Part model, mm, in its own coordinate system. A direction names the side the tool comes from. Round coordinates to 2 decimals unless told otherwise and drop trailing zeros. Write each loop counter-clockwise with the first axis right and the second up, starting at its lowest first coordinate (ties: lowest second). Pieces come first, ordered by that corner, then holes. Notation, with made-up numbers: M 53.25,16 L 91.25,16 A27 cw 91.25,38 Z; hole C 49,-7 d7. An arc over 180 degrees is marked long. Answer as a JSON object with one key per item and string values. Group by question number.
1. Which spindle directions (+Z, -Z, +X, -X, +Y, -Y) get a long thin tool onto all of the face, cutting with end or side? Do faces 1 (the face through (-36, 6.9, 55)), 2 (the face through (36, 3.1, 30)), 3 (the face through (-29.35, 3.25, 41.67)), 4 (the face through (-36, 3.1, 51)). Say none if no direction does.
2. Drill centre lines: line 1 (Z direction, x = -23.5, y = 6.25); line 2 (Y direction, x = -29.5, z = 47); line 3 (X direction, y = 0.75, z = 6). Where is each one in solid material? Low to high. Write a range as from..to.
3. Two-plate mould, pull along Y, no slides. Class faces 5 (the face through (-1, 5, 60)), 6 (the face through (30.301, 7.805, 29.58)), 7 (the face through (-30.552, 2.387, 49.883)): +Y half, -Y half, draft (parallel to the pull), parting line (faces both ways), or undercut.
4. Drop flat-ended pins along their axis: pin 1 (0.5 mm diameter, centred on y = 0.5, z = 45.5, fed in from -X); pin 2 (8 mm diameter, centred on x = 34.5, z = 31.5, fed in from +Y); pin 3 (1.8 mm diameter, centred on x = -32.5, z = 48.5, fed in from +Y). Give the stop position or say it passes through.
5. Band-saw the part on A-A, the plane z = 30.5. Write the cut outline in (x, y), plus the area to 3 significant figures.
6. Band-saw the part on B-B, the plane y = 6. Write the cut outline in (x, z), plus the area to 3 significant figures.
7. Band-saw the part on D-D, the plane z = 53. Write the cut outline in (x, y).
8. Band-saw the part on C-C, the plane x = 34. Write the cut outline in (y, z).
from build123d import *

# Parameters (mm, degrees)
EXTRUDE_1_DEPTH     = 60
CUT_EXTRUDE_1_DEPTH = 17.3


with BuildPart() as part:
    # 스케치1 → 보스-돌출1 (new body)
    with BuildSketch(Plane.XY):
        with BuildLine():
            Line((29.8, 10), (-29.8, 10))
            Line((-29.8, 10), (-29.8, 9.4))
            ThreePointArc((-29.8, 9.4), (-30.532233047, 7.632233047), (-32.3, 6.9))
            Line((-32.3, 6.9), (-39.8, 6.9))
            Line((-39.8, 6.9), (-39.8, 3.1))
            Line((-39.8, 3.1), (-32.3, 3.1))
            ThreePointArc((-32.3, 3.1), (-30.532233047, 2.367766953), (-29.8, 0.6))
            Line((-29.8, 0.6), (-29.8, 0))
            Line((-29.8, 0), (29.8, 0))
            ThreePointArc((29.8, 0), (30.280633401, 2.170456935), (32.3, 3.1))
            Line((32.3, 3.1), (39.8, 3.1))
            Line((39.8, 3.1), (39.8, 6.9))
            Line((39.8, 6.9), (32.3, 6.9))
            ThreePointArc((32.3, 6.9), (30.280633401, 7.829543065), (29.8, 10))
        make_face()
    extrude(amount=EXTRUDE_1_DEPTH)

    # 스케치2 → 컷-돌출1 (cut)
    with BuildSketch(Plane.ZY.offset(39.8)):
        with BuildLine():
            Line((44, 4), (50, 4))
            Line((50, 4), (50, 8))
            Line((50, 8), (10, 8))
            Line((10, 8), (10, 4))
            Line((10, 4), (16, 4))
            ThreePointArc((16, 4), (18.828427125, 2.828427125), (20, 0))
            Line((20, 0), (40, 0))
            ThreePointArc((40, 0), (41.171572875, 2.828427125), (44, 4))
        make_face()
    extrude(amount=-CUT_EXTRUDE_1_DEPTH, mode=Mode.SUBTRACT)


solid = part.part
Worked answers:
{
 "1": {"face 1": "+Z, -Z, -X, +Y", "face 2": "+Z, -Z, +X, -Y", "face 3": "-X", "face 4": "+Z, -Z, -X, -Y"},
 "2": {"line 1": "z = 0..10, 50..60", "line 2": "y = 0..4, 8..10", "line 3": "x = -29.8..29.73"},
 "3": {"face 5": "draft", "face 6": "undercut", "face 7": "-Y half"},
 "4": {"pin 1": "stops at x = -29.8", "pin 2": "stops at y = 7.59", "pin 3": "stops at y = 4"},
 "5": {"outline": "M -30.23,8 L -22.5,8 L -22.5,0 L 29.8,0 A2.5 cw 32.3,3.1 L 39.8,3.1 L 39.8,6.9 L 32.3,6.9 A2.5 cw 29.8,10 L -29.8,10 L -29.8,9.4 A2.5 cw Z", "area": "578 mm^2"},
 "6": {"outline": "M -39.8,0 L 39.8,0 L 39.8,60 L -39.8,60 L -39.8,50 L -22.5,50 L -22.5,10 L -39.8,10 Z", "area": "4,080 mm^2"},
 "7": {"outline": "M -39.8,3.1 L -32.3,3.1 A2.5 cw -29.8,0.6 L -29.8,0 L 29.8,0 A2.5 cw 32.3,3.1 L 39.8,3.1 L 39.8,6.9 L 32.3,6.9 A2.5 cw 29.8,10 L -29.8,10 L -29.8,9.4 A2.5 cw -32.3,6.9 L -39.8,6.9 Z"},
 "8": {"outline": "M 3.1,0 L 6.9,0 L 6.9,60 L 3.1,60 Z"}
}
